Could you check a few things on this model? Use its own coordinates, in mm. Face numbers are marked on the shaded views. A direction names the side the tool comes from. Round coordinates to 2 decimals unless told otherwise and drop trailing zeros. Loops run counter-clockwise (first coordinate to the right, second up) from the corner with the lowest first, then second, coordinate; pieces in that order, holes last. Notation, with made-up numbers: M -6,-31.75 L 13,-31.75 A17 ccw 13,-24.75 Z; hole C 85,-38.5 d1. An arc over 180 degrees is marked long. Answer in a Markdown table with one row per item.
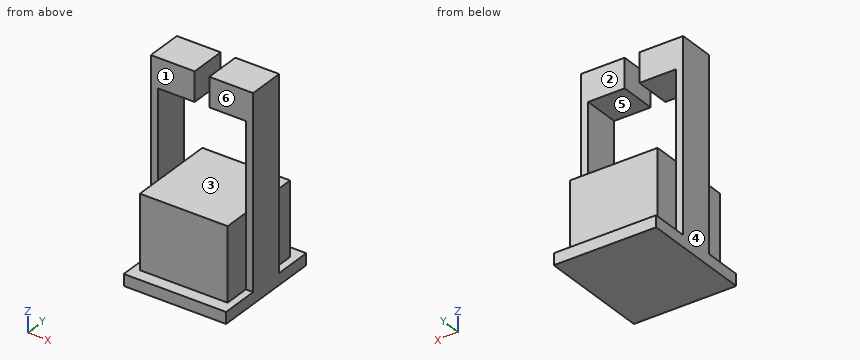
```python
from build123d import *

# Parameters (mm, degrees)
F0_W      = 88.9
F0_H      = 97.79
F1_DEPTH  = 10
F2_W      = 76.2
F2_H      = 76.2
F3_DEPTH  = 63.5
F4_W      = 31.75
F4_H      = 165.1
F5_DEPTH  = 6.35
F6_W      = 31.75
F6_H      = 101.6
F6_H_2    = 63.5
F7_DEPTH  = 6.35
F8_W      = 31.75
F8_H      = 25.4
F9_DEPTH  = 31.75
F10_W     = 31.75
F10_H     = 25.4
F11_DEPTH = 31.75


with BuildPart() as f1:
    # F0 (on Top) → F1 (new body)
    with BuildSketch(Plane.XY):
        with Locations((1.942618, 30.430211)):
            Rectangle(F0_W, F0_H)
    extrude(amount=F1_DEPTH)

    # F2 (on face) → F3 (join)
    with BuildSketch(Plane.XY.offset(10)):
        with Locations((1.942618, 30.430211)):
            Rectangle(F2_W, F2_H)
    extrude(amount=F3_DEPTH)

    # F4 (on face) → F5 (join)
    with BuildSketch(Plane.YZ.offset(40.042618)):
        with Locations((30.430211, 92.55)):
            Rectangle(F4_W, F4_H)
    extrude(amount=F5_DEPTH)

    # F6 (on face) → F7 (join)
    with BuildSketch(Plane(origin=(-36.157382, 0, 0), x_dir=(0, -1, 0), z_dir=(-1, 0, 0))):
        with Locations((-30.430211, 124.3)):
            Rectangle(F6_W, F6_H)
        with Locations((-30.430211, 41.75)):
            Rectangle(F6_W, F6_H_2)
    extrude(amount=F7_DEPTH)

    # F8 (on face) → F9 (join)
    with BuildSketch(Plane(origin=(40.042618, 0, 0), x_dir=(0, -1, 0), z_dir=(-1, 0, 0))):
        with Locations((-30.430211, 162.4)):
            Rectangle(F8_W, F8_H)
    extrude(amount=F9_DEPTH)

    # F10 (on face) → F11 (join)
    with BuildSketch(Plane.YZ.offset(-36.157382)):
        with Locations((30.430211, 162.4)):
            Rectangle(F10_W, F10_H)
    extrude(amount=F11_DEPTH)


solid = f1.part
```
1) I want a section at C-C, the plane y = 20. Please give me the cut outline in (x, z), plus the area to 3 significant figures.
Computed:
| item | result |
|---|---|
| outline | M -42.51,0 L 46.39,0 L 46.39,175.1 L 8.29,175.1 L 8.29,149.7 L 40.04,149.7 L 40.04,73.5 L -36.16,73.5 L -36.16,149.7 L -4.41,149.7 L -4.41,175.1 L -42.51,175.1 Z |
| area | 9,440 mm² |
2) Which directions (+Z, -Z, +X, -X, +Y, -Y) give clear straight access to the entire face, cutting with the end or side of a thin tool? Please do the marked faces 1, 2 and 3.
Computed:
| item | result |
|---|---|
| face 1 | +Z, -X, -Y |
| face 2 | +Z, +X, +Y |
| face 3 | +Y, -Y |
3) If we mould it in two halves opening along X, with no side actions, what happens to the marked faces 4, 5 and 6? For each: released by +X, released by -X, zero draft, split by the parting line, or undercut.
Computed:
| item | result |
|---|---|
| face 4 | released by -X |
| face 5 | undercut |
| face 6 | zero draft |
4) I want a section at B-B, the plane x = 29. Please give me the cut outline in (y, z), plus the area to 3 significant figures.
Computed:
| item | result |
|---|---|
| outline | M -18.46,0 L 79.33,0 L 79.33,10 L 68.53,10 L 68.53,73.5 L -7.67,73.5 L -7.67,10 L -18.46,10 Z; M 14.56,149.7 L 46.31,149.7 L 46.31,175.1 L 14.56,175.1 Z |
| area | 6,620 mm² |
5) Will these pins go through, and if not, where does the flat tip stop? P1, Ø11.5, axis at x = 34.5, z = 56.5, coming from the -Y side; P2, Ø12, axis at y = 59.5, z = 26, coming from the +X side; P3, Ø11, axis at y = 8.5, z = 57.5, coming from the -X side; P4, Ø8, axis at x = 28.5, y = 20.5, coming from the -Z side.
Computed:
| item | result |
|---|---|
| P1 | stops at y = -7.67 |
| P2 | stops at x = 40.04 |
| P3 | stops at x = -36.16 |
| P4 | stops at z = 0 |
6) I need wall thicknesses on line 1 (X direction, y = 36, z = 155); line 2 (Z direction, x = -29, y = 22); line 3 (X direction, y = 22, z = 97.5). Which ranges of each line are inside material? Lowest first, please.
Computed:
| item | result |
|---|---|
| line 1 | x = -42.51 to -4.41, 8.29 to 46.39 |
| line 2 | z = 0 to 73.5, 149.7 to 175.1 |
| line 3 | x = -42.51 to -36.16, 40.04 to 46.39 |
7) I want a section at D-D, the plane x = -1. Please give me the cut outline in (y, z), plus the area to 3 significant figures.
Computed:
| item | result |
|---|---|
| outline | M -18.46,0 L 79.33,0 L 79.33,10 L 68.53,10 L 68.53,73.5 L -7.67,73.5 L -7.67,10 L -18.46,10 Z |
| area | 5,820 mm² |
8) I want a section at A-A, the plane z = 127. Please give me the cut outline in (x, y), plus the area to 3 significant figures.
Computed:
| item | result |
|---|---|
| outline | M -42.51,14.56 L -36.16,14.56 L -36.16,46.31 L -42.51,46.31 Z; M 40.04,14.56 L 46.39,14.56 L 46.39,46.31 L 40.04,46.31 Z |
| area | 403 mm² |
